Autodesk Inventor part; units mm, degrees
ref_plane "YZ Plane" through (0, 0, 0) normal (1, 0, 0) x (0, 1, 0)
ref_plane "XZ Plane" through (0, 0, 0) normal (0, 1, 0) x (-1, 0, 0)
ref_plane "XY Plane" through (0, 0, 0) normal (0, 0, 1) x (1, 0, 0)
sketch "Boceto1" plane through (0, 0, 0) normal (0, 1, 0) x (-1, 0, 0)
  line L0 (10, 66) -> (-10, 66)
  line L1 (-17.5, 58.5) -> (-17.5, -58.5)
  line L2 (-10, -66) -> (10, -66)
  line L3 (17.5, -58.5) -> (17.5, 58.5)
  arc A0 (17.5, 58.5) -> (10, 66) centre (10, 58.5) ccw
  arc A1 (-10, 66) -> (-17.5, 58.5) centre (-10, 58.5) ccw
  arc A2 (-17.5, -58.5) -> (-10, -66) centre (-10, -58.5) ccw
  arc A3 (10, -66) -> (17.5, -58.5) centre (10, -58.5) ccw
  circle A4 centre (-1, 47) radius 9
  circle A5 centre (-1, -16) radius 9
  line L4 (3, 33.5) -> (-5.5, 33.5)
  line L5 (-5.5, 33.5) -> (-5.5, 13.5)
  line L6 (-5.5, 13.5) -> (3, 13.5)
  line L7 (3, 13.5) -> (3, 33.5)
  line L8 (3, -29.5) -> (-5.5, -29.5)
  line L9 (-5.5, -29.5) -> (-5.5, -49.5)
  line L10 (-5.5, -49.5) -> (3, -49.5)
  line L11 (3, -49.5) -> (3, -29.5)
  point P0 (0, 0)
  point P1 (17.5, 66)
  point P2 (-17.5, -66)
  point P3 (17.5, -66)
  point P4 (17.5, 0)
  point P5 (0, -66)
  point P6 (-1.25, 13.5)
  point P7 (-1.25, -49.5)
  point P8 (-1.25, 33.5)
  dimension "d0" = 35
  dimension "d1" = 132
  dimension "d2" = 7.5
  dimension "d5" = 8.5
  dimension "d8" = 20
  dimension "d9" = 12
  dimension "d10" = 43
  dimension "d11" = 16.5
  dimension "d12" = 13.5
  dimension "d13" = 16.5
  dimension "d15" = 18
  dimension "d16" = 13.5
extrude "Extrusión1" add sketch "Boceto1" along normal blind 3
sketch "Boceto2" plane through (0, 0, 0) normal (0, -1, 0) x (1, 0, 0)
  line L0 (17.5, 57) -> (13.5, 57)
  line L1 (13.5, 57) -> (13.5, -57)
  line L2 (13.5, -57) -> (17.5, -57)
  line L3 (17.5, -57) -> (17.5, 57)
  line L4 (-10.5, 57) -> (-13, 57)
  line L5 (-13, 57) -> (-13, -57)
  line L6 (-13, -57) -> (-10.5, -57)
  line L7 (-10.5, -57) -> (-10.5, 57)
  line L8 (16, 57) -> (16, -57)
  line L9 (17.5, 58.5) -> (17.5, -58.5)
  point P0 (0, 0)
  point P1 (17.5, 0)
  point P2 (17.5, 0)
  point P3 (-10.5, 0)
  point P4 (13.5, 0)
  dimension "d19" = 4
  dimension "d20" = 114
  dimension "d21" = 2.5
  dimension "d22" = 2.5
  dimension "d23" = 24
extrude "Extrusión2" add sketch "Boceto2" along normal blind 6.5 contours L8 L2 L1 L0 | L7 L6 L5 L4
extrude "Extrusión3" add sketch "Boceto2" along normal blind 3 contours L3 L2 L8 L0
properties part number "Soporte" material "Plástico ABS"
Could you check a few things on this model? Use its own coordinates, in mm. A direction names the side the tool comes from. Give positions to 0.01 mm unless a question says otherwise; leave off trailing zeros. Order: outer loops, then holes, each group sorted by start corner. A loop starts at its lowest first (then second) coordinate and runs counter-clockwise, first axis right, second up.
Item 1: If we section it at D-D, the plane z = -16: Write out the boundary of the cut face in (x, y).
Item 2: I'm going to push flat-ended pins straight in: pin 1 (2 mm diameter, centred on x = 15.5, y = -4, fed in from -Z); pin 2 (3 mm diameter, centred on y = -4.5, z = 10.5, fed in from -X); pin 3 (11 mm diameter, centred on x = 1, z = -16, fed in from +Y); pin 4 (3 mm diameter, centred on x = -11.5, y = -3.5, fed in from +Z). Where does each tip first touch, or does it pass through?
Item 3: If we mould it in two halves opening along Z, with no side actions, what happens to faces 1 (the face through (0, 3, 1)), 2 (the face through (5.5, 1, 24)), 3 (the face through (15, -3, 57))? For each: pulls with the +Z half, pulls with the -Z half, needs draft (parallel to the pull), parting line crosses it, or undercut.
Item 4: If we section it at B-B, the plane x = 1: Write out the boundary of the cut face in (y, z), plus the area to 3 significant figures.
Item 5: For faces 4 (the face through (16, -5, 1)), 5 (the face through (-12, -3, -57)), 6 (the face through (-3, 1, -40)), 7 (the face through (-10.5, -3, -1)), which set-ups out of +Z, -Z, +X, -X, +Y, -Y let a thin tool reach every point of the face, with its end or its side?
Item 6: If we section it at A-A, the plane z = 25.5: Write out the boundary of the cut face in (x, y).
Item 7: If we section it at C-C, the plane y = 1.75: Write out the boundary of the cut face in (x, z), plus the area to 3 significant figures.
Item 8: I need wall thicknesses on line 1 (Z direction, x = 1, y = 1.35); line 2 (X direction, y = -0.5, z = 53.5); line 3 (X direction, y = -5.75, z = -0.5). Which ranges of each line are inside material? Lowest first, please.
Values:
1. outline: (-17.5, 0) - (-13, 0) - (-13, -6.5) - (-10.5, -6.5) - (-10.5, 0) - (-8, 0) - (-8, 3) - (-17.5, 3) - close; (10, 0) - (13.5, 0) - (13.5, -6.5) - (16, -6.5) - (16, -3) - (17.5, -3) - (17.5, 3) - (10, 3) - close
2. pin 1: stops at z = -57
2. pin 2: stops at x = -13
2. pin 3: passes through
2. pin 4: stops at z = 57
3. face 1: needs draft
3. face 2: undercut
3. face 3: pulls with the +Z half
4. outline: (0, -66) - (3, -66) - (3, -49.5) - (0, -49.5) - close; (0, -29.5) - (3, -29.5) - (3, -25) - (0, -25) - close; (0, -7) - (3, -7) - (3, 13.5) - (0, 13.5) - close; (0, 33.5) - (3, 33.5) - (3, 38) - (0, 38) - close; (0, 56) - (3, 56) - (3, 66) - (0, 66) - close
4. area: 168 mm2
5. face 4: +Z, -Z, +X, -Y
5. face 5: -Z, +X, -X, -Y
5. face 6: +Y, -Y
5. face 7: +Z, -Z, -Y
6. outline: (-17.5, 0) - (-13, 0) - (-13, -6.5) - (-10.5, -6.5) - (-10.5, 0) - (-3, 0) - (-3, 3) - (-17.5, 3) - close; (5.5, 0) - (13.5, 0) - (13.5, -6.5) - (16, -6.5) - (16, -3) - (17.5, -3) - (17.5, 3) - (5.5, 3) - close
7. outline: (-17.5, -58.5) arc R7.5 ccw to (-10, -66) - (10, -66) arc R7.5 ccw to (17.5, -58.5) - (17.5, 58.5) arc R7.5 ccw to (10, 66) - (-10, 66) arc R7.5 ccw to (-17.5, 58.5) - close; hole circle Ø18 at (1, -16); hole circle Ø18 at (1, 47); hole (-3, -49.5) - (5.5, -49.5) - (5.5, -29.5) - (-3, -29.5) - close; hole (-3, 13.5) - (5.5, 13.5) - (5.5, 33.5) - (-3, 33.5) - close
7. area: 3,720 mm2
8. line 1: z = -66 to -49.5, -29.5 to -25, -7 to 13.5, 33.5 to 38, 56 to 66
8. line 2: x = -13 to -10.5, 13.5 to 17.5
8. line 3: x = -13 to -10.5, 13.5 to 16
